For this review, take the finished solid that the model builds, in its own axes (mm). A direction names the side the tool comes from. Give positions to 0.01 mm unless a question says otherwise; leave off trailing zeros. Loops run counter-clockwise (first coordinate to the right, second up) from the corner with the lowest first, then second, coordinate; pieces in that order, holes last. Notation, with made-up numbers: (21.25, 24.5) - (53.25, 24.5) arc R22 cw to (53.25, 48.5) - close; hole circle Ø8 at (15, -22.75). An arc over 180 degrees is marked (long way). Answer as CSV lines item,"result".
from build123d import *

# Parameters (mm, degrees)
SKETCH2_R           = 1.5
BOSS_EXTRUDE1_DEPTH = 3


with BuildPart() as part:
    # Sketch2 → Boss-Extrude1 (new body)
    with BuildSketch(Plane.XY):
        Polygon((0, 6.979195336), (0, -15), (118.208469634, -15), (118.208469634, 115.11627907), (111.041802967, 115.11627907), align=None)
        Polygon((108.208469634, 0), (7.166666667, 0), (108.208469634, 98.398671636), align=None, mode=Mode.SUBTRACT)
        with Locations((107.462245122, 104.651162791)):
            Circle(SKETCH2_R, mode=Mode.SUBTRACT)
        with Locations((10.746224512, 10.465116279)):
            Circle(SKETCH2_R, mode=Mode.SUBTRACT)
        with Locations((110.708469634, -7.5)):
            Circle(SKETCH2_R, mode=Mode.SUBTRACT)
        with Locations((7.5, -7.5)):
            Circle(SKETCH2_R, mode=Mode.SUBTRACT)
        with Locations((59.104234817, -7.5)):
            Circle(SKETCH2_R, mode=Mode.SUBTRACT)
    extrude(amount=BOSS_EXTRUDE1_DEPTH)


solid = part.part
1) Consider section C-C on z = 2. Write out the cut boundary in (x, y).
From the geometry:
outline,"(0, -15) - (118.21, -15) - (118.21, 115.12) - (111.04, 115.12) - (0, 6.98) - close; hole circle Ø3 at (7.5, -7.5); hole (7.17, 0) - (108.21, 0) - (108.21, 98.4) - close; hole circle Ø3 at (10.75, 10.47); hole circle Ø3 at (59.1, -7.5); hole circle Ø3 at (107.46, 104.65); hole circle Ø3 at (110.71, -7.5)"
2) Insertion check: P1, Ø1.5, axis at x = 53, z = 1, coming from the +Y side; P2, Ø1.5, axis at y = 42.5, z = 0.5, coming from the -X side. Each pin has a flat end and moves straight along its axis. Give the tip position at first contact, or say it passes through.
From the geometry:
P1,"stops at y = 59.32"
P2,"stops at x = 35.7"
3) Draft analysis for pull direction Y (two halves, no side actions). For faces 3 (the flat face through (0, -4, 1)), 4 (the flat face through (115, 115.116, 1)), 5 (the flat face through (56.98, 48.51, 1.48)), state which applies: pulls with the +Y half, pulls with the -Y half, needs draft (parallel to the pull), parting line crosses it, or undercut.
From the geometry:
face 3,"needs draft"
face 4,"pulls with the +Y half"
face 5,"undercut"
4) Wall thickness on line 1 (Y direction, x = 9.5, z = 0.35); line 2 (Y direction, x = 7.5, z = 1.9); line 3 (X direction, y = 16, z = 1.55): over which ranges is each line inside the solid? List them lowest first. Write a range as from..to.
From the geometry:
line 1,"y = -15..0, 2.27..9.63, 11.3..16.23"
line 2,"y = -15..-9, -6..0, 0.32..14.28"
line 3,"x = 9.26..23.6, 108.21..118.21"
5) Consider section B-B on x = 33. Write out the cut boundary in (y, z), and give its area (3 significant figures).
From the geometry:
outline,"(-15, 0) - (0, 0) - (0, 3) - (-15, 3) - close; (25.16, 0) - (39.12, 0) - (39.12, 3) - (25.16, 3) - close"
area,"86.9 mm^2"
6) Consider section D-D on y = 85.5. Write out the cut boundary in (x, z), and give its area (3 significant figures).
From the geometry:
outline,"(80.63, 0) - (94.96, 0) - (94.96, 3) - (80.63, 3) - close; (108.21, 0) - (118.21, 0) - (118.21, 3) - (108.21, 3) - close"
area,"73.0 mm^2"
7) Machinability: for faces 1 (the flat face through (108.208, 50, 1)), 2 (the flat face through (58, -15, 1)), which of the approach directions +Z, -Z, +X, -X, +Y, -Y give a long, thin tool a straight path to every point of the face, cutting with its end or side? Answer none if there is none.
From the geometry:
face 1,"+Z, -Z"
face 2,"+Z, -Z, +X, -X, -Y"
8) Consider section A-A on y = -7.5. Write out the cut boundary in (x, z), and give its area (3 significant figures).
From the geometry:
outline,"(0, 0) - (6, 0) - (6, 3) - (0, 3) - close; (9, 0) - (57.6, 0) - (57.6, 3) - (9, 3) - close; (60.6, 0) - (109.21, 0) - (109.21, 3) - (60.6, 3) - close; (112.21, 0) - (118.21, 0) - (118.21, 3) - (112.21, 3) - close"
area,"328 mm^2"
